```python
from build123d import *

# Parameters (mm, degrees)
F0_R           = 75
F1_DEPTH       = 12.7
F2_D           = 5.5
F2_CBORE_D     = 9.75
F2_CBORE_DEPTH = 5
F4_D           = 7
F5_D           = 7.9375
F6_SIZE        = 0.5


# Not quite as in the source:
# - a length typed as a fraction of an inch, garbled in the dataset ("3 / 203.2 mm" for 3/8 in), is restored


with BuildPart() as f1:
    # F0 (on Top) → F1 (new body)
    with BuildSketch(Plane.XY):
        Circle(F0_R)
    extrude(amount=F1_DEPTH)

    # F2 (through all)
    with Locations(Plane(origin=(0, 0, 0), x_dir=(1, 0, 0), z_dir=(0, 0, -1))):
        with Locations((-20.5, -44), (20.5, -44), (-19, 0), (19, 0), (-20.5, 44), (20.5, 44)):
            CounterBoreHole(F2_D / 2, F2_CBORE_D / 2, F2_CBORE_DEPTH)

    # F4 (through all)
    with Locations(Plane.XY.offset(12.7)):
        with Locations((0, 61), (58, 18.8), (-58, 18.8), (-35.8, -49.3), (35.8, -49.3)):
            Hole(F4_D / 2)

    # F5 (through all)
    with Locations(Plane(origin=(0, 0, 0), x_dir=(1, 0, 0), z_dir=(0, 0, -1))):
        with Locations((0, 0)):
            Hole(F5_D / 2)

    # F6
    f6_edges = [f1.edges().sort_by_distance(p)[0] for p in [
        (-75, 0, 0),
        (-39.3, -49.3, 0),
        (-25.375, -44, 0),
        (-23.875, 0, 0),
        (15.625, -44, 0),
        (32.3, -49.3, 0),
        (-3.96875, 0, 0),
        (14.125, 0, 0),
        (-61.5, 18.8, 0),
        (-25.375, 44, 0),
        (54.5, 18.8, 0),
        (15.625, 44, 0),
        (-3.5, 61, 0),
        (-75, 0, 12.7),
        (-39.3, -49.3, 12.7),
        (-23.25, -44, 12.7),
        (-21.75, 0, 12.7),
        (17.75, -44, 12.7),
        (32.3, -49.3, 12.7),
        (-3.96875, 0, 12.7),
        (16.25, 0, 12.7),
        (-61.5, 18.8, 12.7),
        (-23.25, 44, 12.7),
        (54.5, 18.8, 12.7),
        (17.75, 44, 12.7),
        (-3.5, 61, 12.7),
    ]]
    chamfer(f6_edges, length=F6_SIZE)


solid = f1.part
```
Geometry check sheet. Reference: the model listing, model coordinates, mm. A direction names the side the tool comes from. Coordinates: 2 decimals unless noted, no trailing zeros.
Q1. Sectioned sample at A-A on z = 2.25. Give the number of separate pieces and of enclosed holes in the cut face, and give its area (3 significant figures).
Reply:
separate pieces: 1
enclosed holes: 12
area: 17,000 mm2
Q2. Draft check along Y on faces 3 (the face through (15.5, 1, 12.7)), 4 (the face through (-54.503, 18.954, 6.268)). Enter one of: released by +Y, released by -Y, zero draft, split by the parting line, or undercut.
Reply:
face 3: zero draft
face 4: undercut
Q3. Depth check by flat-ended pin: pin 1 Ø5 at (x, y) = (21, -1.5) entering from -Z (3 decimals); pin 2 Ø3 at (y, z) = (-51.5, 4) entering from -X; pin 3 Ø3.5 at (x, y) = (20.5, -44) entering from +Z; pin 4 Ø6 at (x, y) = (20.5, 44) entering from -Z. Enter the tip coordinate at first touch or a pass-through.
Reply:
pin 1: stops at z = 0.375
pin 2: stops at x = -55.9
pin 3: passes through
pin 4: stops at z = 5
Q4. Tool access check on faces 1 (the face through (-21.135, 39.166, 2.718)), 2 (the face through (0.86, 3.874, 6.432)). Record the directions out of +Z, -Z, +X, -X, +Y, -Y that give a thin tool (end or side, any length) a straight path to the whole face; none if there is none.
Reply:
face 1: -Z
face 2: +Z, -Z
Q5. Thickness scan on probe 1 along X at (y, z) = (-44, 2.1) (3 decimals); probe 2 along Y at (x, z) = (19, 3.15) (1 decimal); probe 3 along Y at (x, z) = (20.5, 3.4) (1 decimal). Record the ranges inside material, lowest first.
Reply:
probe 1: x = -60.737 to -25.375, -15.625 to 15.625, 25.375 to 60.737
probe 2: y = -72.6 to -48.6, -39.4 to -4.9, 4.9 to 39.4, 48.6 to 72.6
probe 3: y = -72.1 to -48.9, -39.1 to -4.6, 4.6 to 39.1, 48.9 to 72.1
